Read the model definition and answer for the solid it produces. Units are mm, in the model's axes. Give positions to 0.01 mm unless a question says otherwise; leave off trailing zeros. Write each loop counter-clockwise with the first axis right and the second up, starting at its lowest first coordinate (ties: lowest second). Pieces come first, ordered by that corner, then holes. Notation, with made-up numbers: (-27.5, 43.5) -> (0.5, 43.5) arc R9 cw to (0.5, 57.5) -> close; hole circle Ø10 at (52.25, -40). An arc over 180 degrees is marked (long way). Write item = value, one per line.
from build123d import *

# Parameters (mm, degrees)
F1_DEPTH = 12.7


with BuildPart() as f1:
    # F0 (on Top) → F1 (new body)
    with BuildSketch(Plane.XY):
        with BuildLine():
            ThreePointArc((27.485044, 6.273282), (20.936051, 16.695944), (12.231995, 25.4))
            ThreePointArc((12.231995, 25.4), (0, 26.778215), (-12.231995, 25.4))
            ThreePointArc((-12.231995, 25.4), (-20.936051, 16.695944), (-27.485044, 6.273282))
            ThreePointArc((-27.485044, 6.273282), (-26.106829, -5.958713), (-22.041294, -17.577345))
            ThreePointArc((-22.041294, -17.577345), (-11.618632, -24.126338), (0, -28.191873))
            ThreePointArc((0, -28.191873), (11.618632, -24.126338), (22.041294, -17.577345))
            ThreePointArc((22.041294, -17.577345), (26.106829, -5.958713), (27.485044, 6.273282))
        make_face()
    extrude(amount=F1_DEPTH)


solid = f1.part
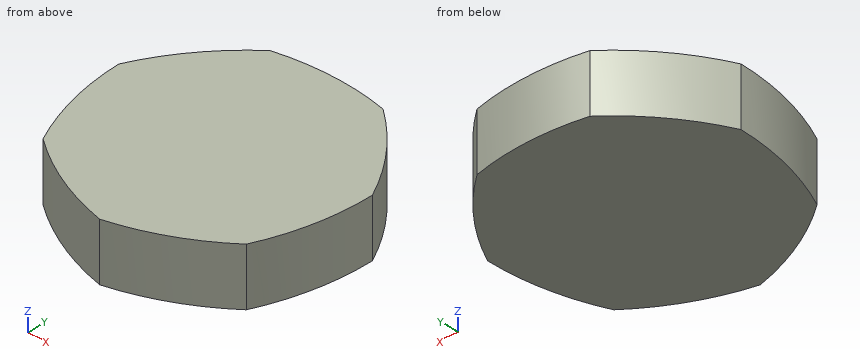
(1) The part is cut by section B-B on y = -24. Determine the outline of the cut face in (x, z), plus the area to 3 significant figures.
Checks:
outline = (-11.88, 0) -> (11.88, 0) -> (11.88, 12.7) -> (-11.88, 12.7) -> close
area = 302 mm²
(2) The part is cut by section C-C on x = -15. Determine the outline of the cut face in (y, z), plus the area to 3 significant figures.
Checks:
outline = (-22.35, 0) -> (23.04, 0) -> (23.04, 12.7) -> (-22.35, 12.7) -> close
area = 576 mm²
(3) Given P1, Ø1.5, axis at y = -7, z = 2, coming from the -X side; P2, Ø3, axis at x = 10, z = 6.5, coming from the -Y side; P3, Ø4, axis at x = 7.5, z = 11, coming from the -Y side, each flat-ended and moving along its own axis, determine where each tip first touches the part or whether it passes through.
Checks:
P1 = -26.04
P2 = -25.51
P3 = -26.63
(4) The part is cut by section A-A on z = 10.5. Determine the outline of the cut face in (x, y).
Checks:
outline = (-27.49, 6.27) arc R54.97 ccw to (-22.04, -17.58) arc R54.97 ccw to (0, -28.19) arc R54.97 ccw to (22.04, -17.58) arc R54.97 ccw to (27.49, 6.27) arc R54.97 ccw to (12.23, 25.4) arc R54.97 ccw to (-12.23, 25.4) arc R54.97 ccw to start
(5) Consider L1, parallel to Y at x = -23, z = 3.75; L2, parallel to X at y = -3, z = 1.75; L3, parallel to X at y = 4.5, z = 6.25. Determine where each line is inside the solid, lowest interval first.
Checks:
L1 = -15.47 to 13.93
L2 = -26.7 to 26.7
L3 = -27.46 to 27.46
